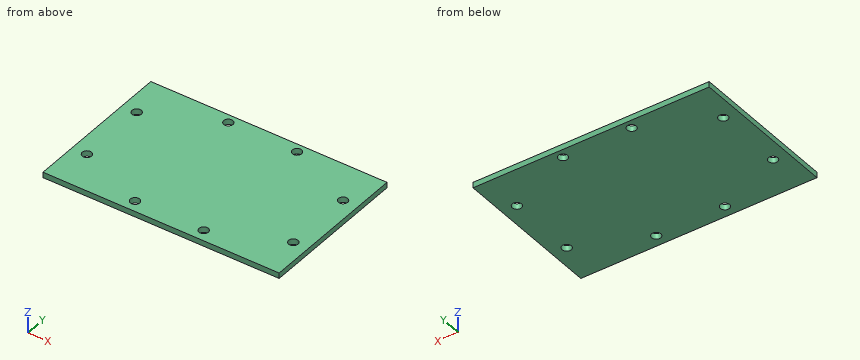
Autodesk Inventor part; units mm, degrees
ref_plane "YZ Plane" through (0, 0, 0) normal (1, 0, 0) x (0, 1, 0)
ref_plane "XZ Plane" through (0, 0, 0) normal (0, 1, 0) x (-1, 0, 0)
ref_plane "XY Plane" through (0, 0, 0) normal (0, 0, 1) x (1, 0, 0)
sketch "Sketch1" plane through (0, 0, 0) normal (0, 0, 1) x (1, 0, 0)
  line L0 (-202.8675, 130) -> (202.8675, 130)
  line L1 (202.8675, 130) -> (202.8675, -130)
  line L2 (202.8675, -130) -> (-202.8675, -130)
  line L3 (-202.8675, -130) -> (-202.8675, 130)
  point P0 (0, 0)
  dimension "d0" = 405.735
  dimension "d1" = 260
  dimension "d2" = 130
  dimension "d3" = 202.8675
extrude "Plate1" add sketch "Sketch1" along normal blind 9.5
sketch "Sketch2" plane through (0, 0, 9.5) normal (0, 0, 1) x (1, 0, 0)
  line L0 (-59, 115) -> (59, 115)
  line L1 (59, 115) -> (59, -110)
  line L2 (59, -110) -> (-59, -110)
  line L3 (-59, -110) -> (-59, 115)
  line L4 (-202.8675, -130) -> (-202.8675, 130)
  line L5 (202.8675, -130) -> (-202.8675, -130)
  line L6 (-177.25, 60) -> (177.25, 60)
  line L7 (177.25, 60) -> (177.25, -60)
  line L8 (177.25, -60) -> (-177.25, -60)
  line L9 (-177.25, -60) -> (-177.25, 60)
  line L10 (202.8675, 130) -> (202.8675, -130)
  point P0 (0, 0)
  dimension "d5" = 118
  dimension "d7" = 225
  dimension "d8" = 20
  dimension "d17" = 120
  dimension "d18" = 60
  dimension "d21" = 118.25
  dimension "d22" = 118.25
  dimension "d23" = 59
hole "Hole1" at (-59, -110, 9.5) at (-59, 115, 9.5) at (59, 115, 9.5) at (59, -110, 9.5) at (-177.25, 60, 9.5) at (-177.25, -60, 9.5) at (177.25, 60, 9.5) at (177.25, -60, 9.5) direction (0, 0, -1) diameter 16 depth 9.5
equation "\"d14\" = Thickness"
equation "\"d4\" = Thickness"
equation "\"BendRadius\" = Thickness"
equation "\"BendReliefWidth\" = Thickness"
equation "\"BendReliefDepth\" = 0.5 * Thickness"
equation "\"CornerReliefSize\" = 4 * Thickness"
equation "\"MinimumRemnant\" = 2 * Thickness"
equation "\"TransitionRadius\" = BendRadius"
equation "\"JacobiRadiusSize\" = BendRadius"
equation "\"GapSize\" = Thickness"
properties part number "PlacaReductor"
Could you check a few things on this model? Use its own coordinates, in mm. Coordinates: 2 decimals unless noted, no trailing zeros. Write each loop counter-clockwise with the first axis right and the second up, starting at its lowest first coordinate (ties: lowest second). Pieces come first, ordered by that corner, then holes. Notation, with made-up numbers: (68, -30) - (78, -30) arc R20 cw to (78, -9) - close; hole circle Ø6 at (41, 26). An arc over 180 degrees is marked (long way). Use a Markdown table: item, result.
Q1. Imagine slicing it at A-A (y = 60). List the corners of the cut face in (x, z) for me, and give its area (3 significant figures).
Geometry check:
| item | result |
|---|---|
| outline | (-202.87, 0) - (-185.25, 0) - (-185.25, 9.5) - (-202.87, 9.5) - close; (-169.25, 0) - (169.25, 0) - (169.25, 9.5) - (-169.25, 9.5) - close; (185.25, 0) - (202.87, 0) - (202.87, 9.5) - (185.25, 9.5) - close |
| area | 3,550 mm2 |
Q2. Please list where these lines run through material, in increasing order: L1, parallel to X at y = -60, z = 5.5; L2, parallel to Y at x = 177.25, z = 3; L3, parallel to Y at x = -59, z = 5.75.
Geometry check:
| item | result |
|---|---|
| L1 | x = -202.87 to -185.25, -169.25 to 169.25, 185.25 to 202.87 |
| L2 | y = -130 to -68, -52 to 52, 68 to 130 |
| L3 | y = -130 to -118, -102 to 107, 123 to 130 |
Q3. Imagine slicing it at B-B (x = 177.25). List the corners of the cut face in (y, z) for me, and give its area (3 significant figures).
Geometry check:
| item | result |
|---|---|
| outline | (-130, 0) - (-68, 0) - (-68, 9.5) - (-130, 9.5) - close; (-52, 0) - (52, 0) - (52, 9.5) - (-52, 9.5) - close; (68, 0) - (130, 0) - (130, 9.5) - (68, 9.5) - close |
| area | 2,170 mm2 |
